Here's how the part is built. I have some questions about the finished solid (model axes, mm). A direction names the side the tool comes from. Round coordinates to 2 decimals unless told otherwise and drop trailing zeros. Write each loop counter-clockwise with the first axis right and the second up, starting at its lowest first coordinate (ties: lowest second). Pieces come first, ordered by that corner, then holes. Notation, with made-up numbers: (-12, 46) -> (28, 46) arc R7 cw to (28, 52) -> close; hole circle Ø3 at (54, -7.5). An arc over 180 degrees is marked (long way). Answer in a Markdown table with one row per item.
from build123d import *

# Parameters (mm, degrees)
F1_DEPTH       = 12.7
F3_DEPTH       = 12.701
F5_D           = 2.54
F5_CSINK_D     = 6.604
F5_CSINK_ANGLE = 90
F6_D           = 5
F6_CSINK_D     = 12
F6_CSINK_ANGLE = 90


with BuildPart() as f1:
    # F0 (on Front) → F1 (new body)
    with BuildSketch(Plane.XZ):
        Polygon((63.5, 38.1), (-63.5, 38.1), (-76.2, 25.4), (-76.2, -38.1), (76.2, -38.1), (76.2, 25.4), align=None)
    extrude(amount=F1_DEPTH)

    # F2 (on face) → F3 (cut, through all)
    with BuildSketch(Plane.XZ.offset(12.7)):
        with BuildLine():
            Line((-46.99, 38.1), (-54.61, 38.1))
            Line((-54.61, 38.1), (-54.61, 25.4))
            ThreePointArc((-54.61, 25.4), (-50.8, 21.59), (-46.99, 25.4))
            Line((-46.99, 25.4), (-46.99, 38.1))
        make_face()
        with BuildLine():
            Line((25.4, 4.7625), (0, 4.7625))
            Line((0, 4.7625), (-25.4, 4.7625))
            ThreePointArc((-25.4, 4.7625), (-30.1625, 0), (-25.4, -4.7625))
            Line((-25.4, -4.7625), (0, -4.7625))
            Line((0, -4.7625), (25.4, -4.7625))
            ThreePointArc((25.4, -4.7625), (30.1625, 0), (25.4, 4.7625))
        make_face()
        with BuildLine():
            Line((54.61, 38.1), (46.99, 38.1))
            Line((46.99, 38.1), (46.99, 25.4))
            ThreePointArc((46.99, 25.4), (50.8, 21.59), (54.61, 25.4))
            Line((54.61, 25.4), (54.61, 38.1))
        make_face()
    extrude(amount=-F3_DEPTH, mode=Mode.SUBTRACT)

    # F5 (through all)
    with Locations(Plane.XZ.offset(12.7)):
        with Locations((-69.85, -12.7), (-50.8, -31.75), (50.8, -31.75), (69.85, -12.7)):
            CounterSinkHole(F5_D / 2, F5_CSINK_D / 2, counter_sink_angle=F5_CSINK_ANGLE)

    # F6 (through all)
    with Locations(Plane.XZ.offset(12.7)):
        with Locations((57.15, -6.35)):
            CounterSinkHole(F6_D / 2, F6_CSINK_D / 2, counter_sink_angle=F6_CSINK_ANGLE)


solid = f1.part
1) Which directions (+Z, -Z, +X, -X, +Y, -Y) give clear straight access to the entire face, cutting with the end or side of a thin tool? Please do faces 4 (the face through (46.99, -6, 32)), 5 (the face through (69.9, -6.3, 31.7)), 6 (the face through (0, -6, -4.762)).
Response:
| item | result |
|---|---|
| face 4 | +Z, +Y, -Y |
| face 5 | +Z, +X, +Y, -Y |
| face 6 | +Y, -Y |
2) I want a section at A-A, the plane y = -4.75. Count the separate pieces of the cut face and the enclosed holes in it, and give its area (3 significant figures).
Response:
| item | result |
|---|---|
| separate pieces | 1 |
| enclosed holes | 6 |
| area | 10,600 mm^2 |
3) I want a section at B-B, the plane z = -6.35. List the corners of the cut face in (x, y) for me.
Response:
| item | result |
|---|---|
| outline | (-76.2, -12.7) -> (51.15, -12.7) -> (54.65, -9.2) -> (54.65, 0) -> (-76.2, 0) -> close; (59.65, -9.2) -> (63.15, -12.7) -> (76.2, -12.7) -> (76.2, 0) -> (59.65, 0) -> close |
4) I need wall thicknesses on line 1 (X direction, y = -3, z = -31.75); line 2 (X direction, y = -4.75, z = -12.7); line 3 (Z direction, x = -50.8, y = -7.25). Which ranges of each line are inside material? Lowest first, please. Write a range as [from, to].
Response:
| item | result |
|---|---|
| line 1 | x = [-76.2, -52.07], [-49.53, 49.53], [52.07, 76.2] |
| line 2 | x = [-76.2, -71.12], [-68.58, 68.58], [71.12, 76.2] |
| line 3 | z = [-38.1, -33.02], [-30.48, 21.59] |
5) We'd pull the mould along X, two halves only. Please class faces 1 (the face through (-1, 0, -8)), 2 (the face through (76.2, -6, -7)), 3 (the face through (30.16, -6.44, -0.1)): +X half, -X half, draft (parallel to the pull), parting line (faces both ways), or undercut.
Response:
| item | result |
|---|---|
| face 1 | draft |
| face 2 | +X half |
| face 3 | undercut |
6) I want a section at C-C, the plane x = 0. List the corners of the cut face in (y, z) for me, and give its area (3 significant figures).
Response:
| item | result |
|---|---|
| outline | (-12.7, -38.1) -> (0, -38.1) -> (0, -4.76) -> (-12.7, -4.76) -> close; (-12.7, 4.76) -> (0, 4.76) -> (0, 38.1) -> (-12.7, 38.1) -> close |
| area | 847 mm^2 |
7) For pin 1 (4 mm diameter, centred on y = -7.5, z = 29.5, fed in from +X); pin 2 (4.5 mm diameter, centred on x = 57.15, z = -6.35, fed in from -Y); pin 3 (3 mm diameter, centred on x = 50.8, z = -31.75, fed in from -Y); pin 4 (8 mm diameter, centred on x = -7, z = -3, fed in from +Y), each with a flat end and sliding along its axis, tell me the tip position at first contact or that it passes through.
Response:
| item | result |
|---|---|
| pin 1 | stops at x = 74.1 |
| pin 2 | passes through |
| pin 3 | stops at y = -10.9 |
| pin 4 | stops at y = 0 |
